Input: part model. Units: mm. Frame: model coordinates. Face numbers are marked on the shaded views. A direction names the side the tool comes from. Round coordinates to 2 decimals unless told otherwise and drop trailing zeros. Loops run counter-clockwise (first coordinate to the right, second up) from the corner with the lowest first, then second, coordinate; pieces in that order, holes last. Notation, with made-up numbers: (88, 23.25) - (120, 23.25) arc R11 cw to (120, 40.25) - close; hole circle Ø9 at (56, 34). An arc over 180 degrees is marked (long way). One line per question, with ' | ' between items. Start each with the question number.
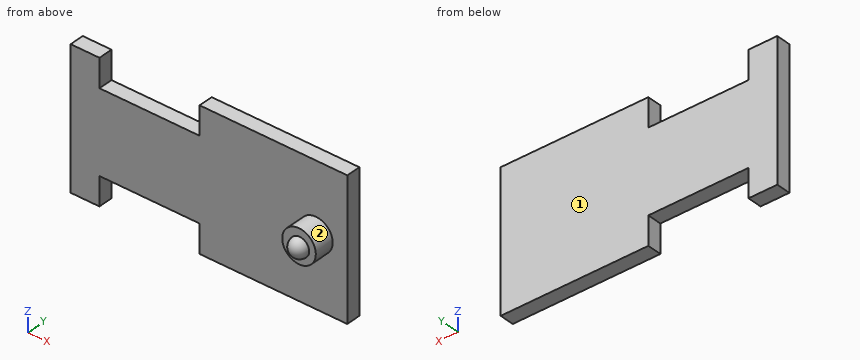
from build123d import *

# Parameters (mm, degrees)
SKETCH1_W           = 101.6
SKETCH1_H           = 50.8
BOSS_EXTRUDE1_DEPTH = 10
SKETCH3_W           = 36.795970914
SKETCH3_H           = 10.40575266
SKETCH3_H_2         = 15.093919488
CUT_EXTRUDE4_DEPTH  = 10
BOSS_EXTRUDE3_DEPTH = 7.412460188
SKETCH8_W           = 111.985504673
SKETCH8_H           = 56.913410447
CUT_EXTRUDE5_DEPTH  = 4.716


with BuildPart() as part:
    # Sketch1 → Boss-Extrude1 (new body)
    with BuildSketch(Plane(origin=(0, 0, 0), x_dir=(1, 0, 0), z_dir=(0, 1, 0))):
        with Locations((-52.916666667, 30.294791667)):
            Rectangle(SKETCH1_W, SKETCH1_H)
    extrude(amount=BOSS_EXTRUDE1_DEPTH)

    # Sketch3 → Cut-Extrude4 (cut)
    with BuildSketch(Plane(origin=(0, 10, 0), x_dir=(1, 0, 0), z_dir=(0, 1, 0))):
        with Locations((-74.746447121, 10.097667997)):
            Rectangle(SKETCH3_W, SKETCH3_H)
        with Locations((-74.746447121, 52.83599875)):
            Rectangle(SKETCH3_W, SKETCH3_H_2)
    extrude(amount=-CUT_EXTRUDE4_DEPTH, mode=Mode.SUBTRACT)

    # Sketch5 → Boss-Extrude3 (add)
    with BuildSketch(Plane.XZ):
        with BuildLine():
            ThreePointArc((-19.801479391, -30.294791667), (-13.631556544, -36.464714513), (-7.461633698, -30.294791667))
            Line((-7.461633698, -30.294791667), (-19.801479391, -30.294791667))
        make_face()
        with BuildLine():
            Line((-19.801479391, -30.294791667), (-7.461633698, -30.294791667))
            ThreePointArc((-7.461633698, -30.294791667), (-13.631556544, -24.12486882), (-19.801479391, -30.294791667))
        make_face()
    extrude(amount=BOSS_EXTRUDE3_DEPTH)

    # Sketch7 → Revolve3 (revolve)
    with BuildSketch(Plane.XZ.offset(7.412460188)):
        with BuildLine():
            Line((-15.363131646, -27.535093848), (-11.467087667, -33.379159817))
            ThreePointArc((-11.467087667, -33.379159817), (-10.493076672, -28.509104843), (-15.363131646, -27.535093848))
        make_face()
    revolve(axis=Axis((-15.363131646, -7.412460188, -27.535093848), (0.5547001962252264, 0, -0.8320502943378455)))

    # Sketch8 → Cut-Extrude5 (cut)
    with BuildSketch(Plane(origin=(0, 10, 0), x_dir=(1, 0, 0), z_dir=(0, 1, 0))):
        with Locations((-50.660840015, 30.234288396)):
            Rectangle(SKETCH8_W, SKETCH8_H)
    extrude(amount=-CUT_EXTRUDE5_DEPTH, mode=Mode.SUBTRACT)


solid = part.part
(1) Section D-D, the plane x = -48.5. Output: boundary loops of the cut face in (y, z), plus the area to 3 significant figures.
(2) Section A-A, the plane z = -13. Output: boundary loops of the cut face in (x, y), plus the area to 3 significant figures.
(3) Section B-B, the plane x = -63.5. Output: boundary loops of the cut face in (y, z).
(4) Pin query (flat end, axial travel): P1, Ø2, axis at x = -48.5, z = -28.5, coming from the -Y side; P2, Ø2.5, axis at x = -69, y = 1.5, coming from the -Z side; P3, Ø2.5, axis at x = -79.5, y = 3.5, coming from the +Z side. Return the tip coordinate at first contact, or that it passes through.
(5) Line query: line 1 along X through (y, z) = (2.75, -12); line 2 along Y through (x, z) = (-10, -49.5); line 3 along Z through (x, y) = (-61.5, 1.75). Output: solid intervals per line, ascending. Write a range as from..to.
(6) Section C-C, the plane y = -9.5. Output: boundary loops of the cut face in (x, z).
(7) Reachability of the marked faces 1 and 2 from +Z, -Z, +X, -X, +Y, -Y: full face, straight path, thin tool, end or side. Return the list, or none.
Derived:
1) outline: (0, -55.69) - (5.28, -55.69) - (5.28, -4.89) - (0, -4.89) - close | area: 268 mm²
2) outline: (-103.72, 0) - (-93.14, 0) - (-93.14, 5.28) - (-103.72, 5.28) - close; (-56.35, 0) - (-2.12, 0) - (-2.12, 5.28) - (-56.35, 5.28) - close | area: 342 mm²
3) outline: (0, -45.29) - (5.28, -45.29) - (5.28, -15.3) - (0, -15.3) - close
4) P1: stops at y = 0 | P2: stops at z = -45.29 | P3: stops at z = -15.3
5) line 1: x = -103.72..-93.14, -56.35..-2.12 | line 2: y = 0..5.28 | line 3: z = -45.29..-15.3
6) outline: circle Ø5.65 at (-13.42, -30.46)
7) face 1: +Z, -Z, +X, -X, +Y | face 2: -Y
